from build123d import *

# Parameters (mm, degrees)
ESQUISSE1_R        = 1.5
BOSS_EXTRU_1_DEPTH = 5


with BuildPart() as part:
    # Esquisse1 → Boss.-Extru.1 (new body)
    with BuildSketch(Plane(origin=(0, 0, 0), x_dir=(1, 0, 0), z_dir=(0, 1, 0))):
        with BuildLine():
            Line((40.864149318, 35.778782826), (53.139812779, 57.040855637))
            ThreePointArc((53.139812779, 57.040855637), (54.138817004, 64.629046088), (49.479558741, 70.701109675))
            Line((49.479558741, 70.701109675), (36.489177684, 78.201109675))
            ThreePointArc((36.489177684, 78.201109675), (28.900987233, 79.2001139), (22.828923646, 74.540855637))
            Line((22.828923646, 74.540855637), (10.553260185, 53.278782826))
            ThreePointArc((10.553260185, 53.278782826), (2.360755727, 44.121425984), (-8.815715388, 39.016447329))
            ThreePointArc((-8.815715388, 39.016447329), (-20, 34.641016151), (-29.381376859, 27.142857143))
            ThreePointArc((-29.381376859, 27.142857143), (-39.390653617, 20.016238561), (-51.417409503, 17.5))
            Line((-51.417409503, 17.5), (-75.968736425, 17.5))
            ThreePointArc((-75.968736425, 17.5), (-83.039804237, 14.571067812), (-85.968736425, 7.5))
            Line((-85.968736425, 7.5), (-85.968736425, -7.5))
            ThreePointArc((-85.968736425, -7.5), (-83.039804237, -14.571067812), (-75.968736425, -17.5))
            Line((-75.968736425, -17.5), (-51.417409503, -17.5))
            ThreePointArc((-51.417409503, -17.5), (-39.390653617, -20.016238561), (-29.381376859, -27.142857143))
            ThreePointArc((-29.381376859, -27.142857143), (-20, -34.641016151), (-8.815715388, -39.016447329))
            ThreePointArc((-8.815715388, -39.016447329), (2.360755727, -44.121425984), (10.553260185, -53.278782826))
            Line((10.553260185, -53.278782826), (22.828923646, -74.540855637))
            ThreePointArc((22.828923646, -74.540855637), (28.900987233, -79.2001139), (36.489177684, -78.201109675))
            Line((36.489177684, -78.201109675), (49.479558741, -70.701109675))
            ThreePointArc((49.479558741, -70.701109675), (54.138817004, -64.629046088), (53.139812779, -57.040855637))
            Line((53.139812779, -57.040855637), (40.864149318, -35.778782826))
            ThreePointArc((40.864149318, -35.778782826), (37.02989789, -24.105187424), (38.197092246, -11.873590187))
            ThreePointArc((38.197092246, -11.873590187), (40, 0), (38.197092246, 11.873590187))
            ThreePointArc((38.197092246, 11.873590187), (37.02989789, 24.105187424), (40.864149318, 35.778782826))
        make_face()
        with Locations(Location((-75.968736425, 2.5, 0), (0, 0, 270))):
            Circle(ESQUISSE1_R, mode=Mode.SUBTRACT)
        with Locations(Location((-45.968736425, 2.5, 0), (0, 0, 270))):
            Circle(ESQUISSE1_R, mode=Mode.SUBTRACT)
        with Locations(Location((40.149431722, 64.540855637, 0), (0, 0, 270))):
            Circle(ESQUISSE1_R, mode=Mode.SUBTRACT)
        with Locations(Location((25.149431722, 38.560093524, 0), (0, 0, 270))):
            Circle(ESQUISSE1_R, mode=Mode.SUBTRACT)
        with Locations(Location((35.819304703, -67.040855637, 0), (0, 0, 270))):
            Circle(ESQUISSE1_R, mode=Mode.SUBTRACT)
        with Locations(Location((20.819304703, -41.060093524, 0), (0, 0, 270))):
            Circle(ESQUISSE1_R, mode=Mode.SUBTRACT)
    extrude(amount=BOSS_EXTRU_1_DEPTH)


solid = part.part
Design review of the part built by this model. Coordinates are the model's own, in mm. A direction names the side the tool comes from. Coordinates: 2 decimals unless noted, no trailing zeros. Loops run counter-clockwise (first coordinate to the right, second up) from the corner with the lowest first, then second, coordinate; pieces in that order, holes last. Notation, with made-up numbers: (83.25, 38) - (113.25, 38) arc R21 ccw to (113.25, 63) - close; hole circle Ø9 at (-39.75, 65). An arc over 180 degrees is marked (long way). Use CSV: the item, a comma, the result in double quotes. Start each with the question number.
1. Mouldability with a two-part tool opening along Z and no side actions: class faces 3 (the cylindrical face through (37.05, 2.46, 24.28)), 4 (the cylindrical face through (28.79, 2.46, 79.17)), 5 (the cylindrical face through (29.01, 2.46, -79.23)) as released by +Z, released by -Z, zero draft, split by the parting line, or undercut.
2. Add section C-C on z = -33.5. Give the boundary of the cut face in (x, y).
3. Add section B-B on x = -68. Give the boundary of the cut face in (y, z).
4. Add section A-A on y = 3.15. Count the separate pieces of the cut face and the enclosed holes in it, plus the area to 3 significant figures.
5. For faces 1 (the flat face through (-64, 2, 17.5)), 2 (the cylindrical face through (54.167, 2.465, -64.523)), list the 3-axis set-ups (+Z, -Z, +X, -X, +Y, -Y) from which the entire face can be reached by the end or side of a thin tool; tool diameter is ignored.
6. Clearance check with flat-ended pins moving along their axes: pin 1 (2.5 mm diameter, centred on x = -65, y = 2.5, fed in from +Z); pin 2 (3 mm diameter, centred on x = -46.5, y = 1, fed in from -Z); pin 3 (2.5 mm diameter, centred on x = 40.15, z = -64.54, fed in from +Y); pin 4 (1.5 mm diameter, centred on y = 2, z = -33.5, fed in from +X). State where each tip first meets the part, or that it passes through.
7. To check wall thickness, follow probe 1 along X at (y, z) = (1.3, -2); probe 2 along Z at (x, y) = (-67.5, 0.7); probe 3 along X at (y, z) = (2.6, -2.5). State the ranges of each line that lie inside material, in increasing order.
Resolved:
1,face 3,"undercut"
1,face 4,"released by +Z"
1,face 5,"released by -Z"
2,outline,"(-21.86, 0) - (39.68, 0) - (39.68, 5) - (-21.86, 5) - close"
3,outline,"(0, -17.5) - (5, -17.5) - (5, 17.5) - (0, 17.5) - close"
4,separate pieces,"1"
4,enclosed holes,"6"
4,area,"10,000 mm2"
5,face 1,"+Z, -X, +Y, -Y"
5,face 2,"+X, +Y, -Y"
6,pin 1,"z = 17.5"
6,pin 2,"z = -18.19"
6,pin 3,"through"
6,pin 4,"x = 40.04"
7,probe 1,"-85.97 to -77.38, -74.55 to -47.38, -44.55 to 39.95"
7,probe 2,"-17.5 to 17.5"
7,probe 3,"-85.97 to -77.47, -74.47 to -47.47, -44.47 to 39.92"
